For this review, take the finished solid that the model builds, in its own axes (mm). A direction names the side the tool comes from. Coordinates: 2 decimals unless noted, no trailing zeros. Order: outer loops, then holes, each group sorted by start corner. A loop starts at its lowest first (then second) coordinate and runs counter-clockwise, first axis right, second up. Notation, with made-up numbers: M 0,-25.75 L 37,-25.75 A11 cw 37,-15.75 Z; hole C -23.75,84.5 d4. An arc over 180 degrees is marked long. Use CSV: the item, a comma, the result in double quotes.
```python
from build123d import *

# Parameters (mm, degrees)
F0_R     = 9.5
F1_DEPTH = 10


with BuildPart() as f1:
    # F0 (on Top) → F1 (new body)
    with BuildSketch(Plane.XY):
        with BuildLine():
            ThreePointArc((-45.603654, 15.217773), (-46.480887, 16.137107), (-47.551994, 15.45341))
            ThreePointArc((-47.551994, 15.45341), (-49.992271, -0.879128), (-46.979256, -17.115769))
            ThreePointArc((-46.979256, -17.115769), (-41.501628, -25.193784), (-32.853296, -29.717619))
            ThreePointArc((-32.853296, -29.717619), (-29.737157, -30.296193), (-26.577854, -30.548923))
            ThreePointArc((-26.577854, -30.548923), (-19.287217, -28.888307), (-13.704095, -23.914398))
            ThreePointArc((-13.704095, -23.914398), (-7.766577, -18.516867), (0, -16.5))
            ThreePointArc((0, -16.5), (16.184433, -28.225238), (9.622849, -47.102809))
            ThreePointArc((9.622849, -47.102809), (9.265298, -48.322182), (10.392951, -48.90794))
            ThreePointArc((10.392951, -48.90794), (25.757483, -42.855012), (38.312318, -32.127345))
            ThreePointArc((38.312318, -32.127345), (42.569271, -23.344572), (42.162861, -13.592979))
            ThreePointArc((42.162861, -13.592979), (41.105851, -10.605037), (39.74507, -7.742635))
            ThreePointArc((39.74507, -7.742635), (34.661617, -2.259066), (27.562523, 0.089105))
            ThreePointArc((27.562523, 0.089105), (12.499757, 21.089495), (35.980805, 31.885036))
            ThreePointArc((35.980805, 31.885036), (37.215588, 32.185075), (37.159042, 33.45453))
            ThreePointArc((37.159042, 33.45453), (24.234788, 43.734141), (8.666937, 49.243113))
            ThreePointArc((8.666937, 49.243113), (-1.067643, 48.538356), (-9.309565, 43.310599))
            ThreePointArc((-9.309565, 43.310599), (-11.368694, 40.90123), (-13.167216, 38.291558))
            ThreePointArc((-13.167216, 38.291558), (-15.3744, 31.147374), (-13.858429, 23.825293))
            ThreePointArc((-13.858429, 23.825293), (-24.513917, 0.280359), (-45.603654, 15.217773))
        make_face()
        with Locations((-25.980762, -15)):
            Circle(F0_R, mode=Mode.SUBTRACT)
        Circle(F0_R, mode=Mode.SUBTRACT)
        with Locations((25.980762, -15)):
            Circle(F0_R, mode=Mode.SUBTRACT)
        with Locations((0, 30)):
            Circle(F0_R, mode=Mode.SUBTRACT)
    extrude(amount=F1_DEPTH)


solid = f1.part
```
Item 1: To check wall thickness, follow line 1 along Y through (x, z) = (-8.5, 0.75); line 2 along Y through (x, z) = (26, 5); line 3 along X through (y, z) = (5, 8). State the ranges of each line that lie inside material, in increasing order. Write a range as [from, to].
Solutions:
line 1,"[-18.94, -4.24], [4.24, 25.76], [34.24, 44.12]"
line 2,"[-42.71, -24.5], [-5.5, 0.27], [33.34, 42.71]"
line 3,"[-49.75, -41.13], [-16.67, -8.08], [8.08, 16.81]"
Item 2: For faces 4 (the face through (-19.381, -28.936, 4.93)), 5 (the face through (12.4, 20.7, 4.9)), 6 (the face through (34.75, -2.317, 4.93)), list the 3-axis set-ups (+Z, -Z, +X, -X, +Y, -Y) from which the entire face can be reached by the end or side of a thin tool; tool diameter is ignored.
Solutions:
face 4,"+Z, -Z, -Y"
face 5,"+Z, -Z"
face 6,"+Z, -Z, +X"
Item 3: Clearance check with flat-ended pins moving along their axes: pin 1 Ø5 at (y, z) = (39.5, 2) entering from -X; pin 2 Ø2 at (x, z) = (17, 1.5) entering from +Y; pin 3 Ø1 at (x, z) = (-37, 4) entering from +Y; pin 4 Ø5 at (x, y) = (14, 17) entering from -Z. State where each tip first meets the part, or that it passes through.
Solutions:
pin 1,"x = -13.88"
pin 2,"y = 47.37"
pin 3,"y = 2.07"
pin 4,"z = 0"
Item 4: Add section C-C on y = -22. State the section outline as (x, z) points.
Solutions:
outline,"M -44.39,0 L -32.4,0 L -32.4,10 L -44.39,10 Z; M -19.56,0 L -12.21,0 L -12.21,10 L -19.56,10 Z; M 12.62,0 L 19.56,0 L 19.56,10 L 12.62,10 Z; M 32.4,0 L 42.8,0 L 42.8,10 L 32.4,10 Z"
Item 5: Draft analysis for pull direction X (two halves, no side actions). For faces 1 (the face through (-15.37, 31.25, 4.93)), 2 (the face through (-4, -10, 10)), 3 (the face through (-24.1, 0.4, 4.9)), state which applies: released by +X, released by -X, zero draft, split by the parting line, or undercut.
Solutions:
face 1,"released by -X"
face 2,"zero draft"
face 3,"undercut"
Item 6: Add section A-A on x = 22.5. State the section outline as (y, z) points, and give its area (3 significant figures).
Solutions:
outline,"M -44.65,0 L -23.84,0 L -23.84,10 L -44.65,10 Z; M -6.16,0 L 1.24,0 L 1.24,10 L -6.16,10 Z; M 32.37,0 L 44.65,0 L 44.65,10 L 32.37,10 Z"
area,"405 mm^2"
Item 7: Add section D-D on z = 4.5. State the section outline as (x, y) points, and give its area (3 significant figures).
Solutions:
outline,"M -47.55,15.45 A50 ccw -46.98,-17.12 A20 ccw -32.85,-29.72 A30.56 ccw -26.58,-30.55 A15 ccw -13.7,-23.91 A16.75 cw long 9.62,-47.1 A1 ccw 10.39,-48.91 A50 ccw 38.31,-32.13 A20 ccw 42.16,-13.59 A30.56 ccw 39.75,-7.74 A15 ccw 27.56,0.09 A16.75 cw long 35.98,31.89 A1 ccw 37.16,33.45 A50 ccw 8.67,49.24 A20 ccw -9.31,43.31 A30.56 ccw -13.17,38.29 A15 ccw -13.86,23.83 A16.75 cw long -45.6,15.22 A1 ccw Z; hole C -25.98,-15 d19; hole C 0,0 d19; hole C 0,30 d19; hole C 25.98,-15 d19"
area,"3,100 mm^2"
Item 8: Add section B-B on y = 37. State the section outline as (x, z) points, and give its area (3 significant figures).
Solutions:
outline,"M -13.88,0 L -6.42,0 L -6.42,10 L -13.88,10 Z; M 6.42,0 L 33.63,0 L 33.63,10 L 6.42,10 Z"
area,"347 mm^2"
